Part model, mm, in its own coordinate system. A direction names the side the tool comes from. Give positions to 0.01 mm unless a question says otherwise; leave off trailing zeros. Write each loop counter-clockwise with the first axis right and the second up, starting at its lowest first coordinate (ties: lowest second). Pieces come first, ordered by that corner, then holes.
from build123d import *

# Parameters (mm, degrees)
BOSS_EXTRUDE1_DEPTH = 250


with BuildPart() as part:
    # Sketch1 → Boss-Extrude1 (new body)
    with BuildSketch(Plane.XY):
        with BuildLine():
            Line((-20, -25), (-7.464101615, -25))
            Line((-7.464101615, -25), (-4, -19))
            Line((-4, -19), (4, -19))
            Line((4, -19), (7.464101615, -25))
            Line((7.464101615, -25), (20, -25))
            Line((20, -25), (20, -20))
            Line((20, -20), (9.25, -20))
            Line((9.25, -20), (3.75, -7.066647013))
            ThreePointArc((3.75, -7.066647013), (0, -8), (-3.75, -7.066647013))
            Line((-3.75, -7.066647013), (-9.25, -20))
            Line((-9.25, -20), (-20, -20))
            Line((-20, -20), (-20, -25))
        make_face()
    extrude(amount=BOSS_EXTRUDE1_DEPTH)


solid = part.part
1) Flat gauge pins, fed straight in: P1, Ø9, axis at x = 0, z = 135, coming from the -Y side; P2, Ø10, axis at x = 7, y = -10, coming from the +Z side; P3, Ø6, axis at y = -9, z = 103, coming from the -X side; P4, Ø1, axis at y = -18.5, z = 67, coming from the -X side. Where does each tip first touch, or does it go through?
Check result:
P1: stops at y = -19.87
P2: stops at z = 250
P3: stops at x = -5.85
P4: stops at x = -8.82
2) Mould opens along X. For faces 1 (the flat face through (14, -25, 123)), 2 (the cylindrical face through (0, -8, 123)), 3 (the flat face through (-6.46, -13.44, 123.25)) say: +X half, -X half, draft (parallel to the pull), parting line (faces both ways), or undercut.
Check result:
face 1: draft
face 2: undercut
face 3: -X half
3) Saw through at B-B (x = -15.5). Write the cut outline in (y, z).
Check result:
outline: (-25, 0) - (-20, 0) - (-20, 250) - (-25, 250) - close
4) Saw through at C-C (y = -10.5). Write the cut outline in (x, z), and give its area (3 significant figures).
Check result:
outline: (-5.21, 0) - (5.21, 0) - (5.21, 250) - (-5.21, 250) - close
area: 2,610 mm2
5) Drill centre lines: L1, parallel to Y at x = 18, z = 20; L2, parallel to Y at x = -3, z = 87; L3, parallel to X at y = -11.75, z = 80.5. Where is each one in solid material? Low to high.
Check result:
L1: y = -25 to -20
L2: y = -19 to -7.42
L3: x = -5.74 to 5.74
6) 3-axis set-ups, long thin cutter, end or side, ignore diameter. For faces 4 (the flat face through (-15, -20, 123)), 5 (the flat face through (-14, -25, 123)), 6 (the flat face through (20, -23, 123)), 7 (the flat face through (15, -20, 123)), 8 (the flat face through (0, -19, 123)): which of +Z, -Z, +X, -X, +Y, -Y reach the whole face in a straight line?
Check result:
face 4: +Z, -Z, -X, +Y
face 5: +Z, -Z, +X, -X, -Y
face 6: +Z, -Z, +X, +Y, -Y
face 7: +Z, -Z, +X, +Y
face 8: +Z, -Z, -Y
7) Saw through at A-A (z = 51.5). Write the cut outline in (x, y), and give its area (3 significant figures).
Check result:
outline: (-20, -25) - (-7.46, -25) - (-4, -19) - (4, -19) - (7.46, -25) - (20, -25) - (20, -20) - (9.25, -20) - (3.75, -7.07) arc R8 cw to (-3.75, -7.07) - (-9.25, -20) - (-20, -20) - close
area: 295 mm2
